```python
from build123d import *

# Parameters (mm, degrees)
SKETCH_1_W          = 35
SKETCH_1_H          = 35
EXTRUDE_1_DEPTH     = 1.6
EXTRUDE_1_2_DEPTH   = 1.6
EXTRUDE_1_3_DEPTH   = 1.6
EXTRUDE_1_4_DEPTH   = 1.6
SKETCH_2_W          = 10
SKETCH_2_H          = 4
SKETCH_2_W_2        = 4
SKETCH_2_H_2        = 10
EXTRUDE_2_DEPTH     = 1.6
CHAMFER_1_SIZE      = 5
FILLET_1_R          = 1
FILLET_2_R          = 2
SKETCH_3_R          = 0.75
CUT_EXTRUDE_1_DEPTH = 105.664033937
SKETCH_4_R          = 0.75
CUT_EXTRUDE_2_DEPTH = 105.664033937


with BuildPart() as part:
    # Sketch 1 → Extrude 1 (new body)
    with BuildSketch(Plane(origin=(0, 0, 0), x_dir=(1, 0, 0), z_dir=(0, 1, 0))):
        with Locations((56.5, -17.5)):
            Rectangle(SKETCH_1_W, SKETCH_1_H)
    extrude(amount=EXTRUDE_1_DEPTH)



with BuildPart() as body_2:
    # Sketch 1 → Extrude 1 2 (new body)
    with BuildSketch(Plane(origin=(0, 0, 0), x_dir=(1, 0, 0), z_dir=(0, 1, 0))):
        with Locations((17.5, -17.5)):
            Rectangle(SKETCH_1_W, SKETCH_1_H)
    extrude(amount=EXTRUDE_1_2_DEPTH)


with BuildPart() as body_3:
    # Sketch 1 → Extrude 1 3 (new body)
    with BuildSketch(Plane(origin=(0, 0, 0), x_dir=(1, 0, 0), z_dir=(0, 1, 0))):
        with Locations((17.5, -56.5)):
            Rectangle(SKETCH_1_W, SKETCH_1_H)
    extrude(amount=EXTRUDE_1_3_DEPTH)


with BuildPart() as body_4:
    # Sketch 1 → Extrude 1 4 (new body)
    with BuildSketch(Plane(origin=(0, 0, 0), x_dir=(1, 0, 0), z_dir=(0, 1, 0))):
        with Locations((56.5, -56.5)):
            Rectangle(SKETCH_1_W, SKETCH_1_H)
    extrude(amount=EXTRUDE_1_4_DEPTH)


with BuildPart() as part_1:
    add(part.part)

    add(body_2.part)  # Extrude 2 merges body 2

    add(body_3.part)  # Extrude 2 merges body 3

    add(body_4.part)  # Extrude 2 merges body 4
    # Sketch 2 → Extrude 2 (add)
    with BuildSketch(Plane(origin=(0, 1.6, 0), x_dir=(1, 0, 0), z_dir=(0, 1, 0))):
        with Locations((15, -37)):
            Rectangle(SKETCH_2_W, SKETCH_2_H)
        with Locations((37, -15)):
            Rectangle(SKETCH_2_W_2, SKETCH_2_H_2)
        with Locations((59, -37)):
            Rectangle(SKETCH_2_W, SKETCH_2_H)
        with Locations((37, -59)):
            Rectangle(SKETCH_2_W_2, SKETCH_2_H_2)
    extrude(amount=-EXTRUDE_2_DEPTH)

    # Chamfer 1
    chamfer_1_edges = [part_1.edges().sort_by_distance(p)[0] for p in [
        (0, 0.8, 39),
        (39, 0.8, 0),
        (39, 0.8, 39),
        (0, 0.8, 0),
    ]]
    chamfer(chamfer_1_edges, length=CHAMFER_1_SIZE)

    # Fillet 1
    fillet_1_edges = [part_1.edges().sort_by_distance(p)[0] for p in [
        (44, 0.8, 39),
        (0, 0.8, 44),
        (5, 0.8, 39),
        (39, 0.8, 5),
        (44, 0.8, 0),
        (0, 0.8, 5),
        (5, 0.8, 0),
        (39, 0.8, 44),
    ]]
    fillet(fillet_1_edges, radius=FILLET_1_R)

    # Fillet 2
    fillet_2_edges = [part_1.edges().sort_by_distance(p)[0] for p in [
        (35, 0.8, 39),
        (0, 0.8, 74),
        (35, 0.8, 74),
        (39, 0.8, 35),
        (74, 0.8, 35),
        (74, 0.8, 0),
        (39, 0.8, 74),
        (74, 0.8, 74),
        (74, 0.8, 39),
        (35, 0.8, 0),
        (35, 0.8, 35),
        (0, 0.8, 35),
    ]]
    fillet(fillet_2_edges, radius=FILLET_2_R)

    # Sketch 3 → Cut-Extrude 1 (cut, through all)
    with BuildSketch(Plane(origin=(0, 1.6, 0), x_dir=(1, 0, 0), z_dir=(0, 1, 0))):
        with Locations(Location((11, -35.5, 0), (0, 0, 270))):
            Circle(SKETCH_3_R)
        with Locations(Location((63, -35.5, 0), (0, 0, 270))):
            Circle(SKETCH_3_R)
        with Locations(Location((63, -38.5, 0), (0, 0, 90))):
            Circle(SKETCH_3_R)
        with Locations(Location((11, -38.5, 0), (0, 0, 90))):
            Circle(SKETCH_3_R)
        with Locations(Location((13, -38.5, 0), (0, 0, 90))):
            Circle(SKETCH_3_R)
        with Locations(Location((13, -35.5, 0), (0, 0, 270))):
            Circle(SKETCH_3_R)
        with Locations(Location((15, -38.5, 0), (0, 0, 90))):
            Circle(SKETCH_3_R)
        with Locations(Location((15, -35.5, 0), (0, 0, 270))):
            Circle(SKETCH_3_R)
        with Locations(Location((17, -38.5, 0), (0, 0, 90))):
            Circle(SKETCH_3_R)
        with Locations(Location((17, -35.5, 0), (0, 0, 270))):
            Circle(SKETCH_3_R)
        with Locations(Location((19, -38.5, 0), (0, 0, 90))):
            Circle(SKETCH_3_R)
        with Locations(Location((19, -35.5, 0), (0, 0, 270))):
            Circle(SKETCH_3_R)
        with Locations(Location((61, -35.5, 0), (0, 0, 270))):
            Circle(SKETCH_3_R)
        with Locations(Location((61, -38.5, 0), (0, 0, 90))):
            Circle(SKETCH_3_R)
        with Locations(Location((59, -35.5, 0), (0, 0, 270))):
            Circle(SKETCH_3_R)
        with Locations(Location((59, -38.5, 0), (0, 0, 90))):
            Circle(SKETCH_3_R)
        with Locations(Location((57, -35.5, 0), (0, 0, 270))):
            Circle(SKETCH_3_R)
        with Locations(Location((57, -38.5, 0), (0, 0, 90))):
            Circle(SKETCH_3_R)
        with Locations(Location((55, -35.5, 0), (0, 0, 270))):
            Circle(SKETCH_3_R)
        with Locations(Location((55, -38.5, 0), (0, 0, 90))):
            Circle(SKETCH_3_R)
    extrude(amount=-CUT_EXTRUDE_1_DEPTH, mode=Mode.SUBTRACT)

    # Sketch 4 → Cut-Extrude 2 (cut, through all)
    with BuildSketch(Plane(origin=(0, 1.6, 0), x_dir=(1, 0, 0), z_dir=(0, 1, 0))):
        with Locations(Location((35.5, -11, 0), (0, 0, 270))):
            Circle(SKETCH_4_R)
        with Locations(Location((38.5, -11, 0), (0, 0, 270))):
            Circle(SKETCH_4_R)
        with Locations(Location((35.5, -13, 0), (0, 0, 270))):
            Circle(SKETCH_4_R)
        with Locations(Location((38.5, -13, 0), (0, 0, 270))):
            Circle(SKETCH_4_R)
        with Locations(Location((35.5, -15, 0), (0, 0, 270))):
            Circle(SKETCH_4_R)
        with Locations(Location((38.5, -15, 0), (0, 0, 270))):
            Circle(SKETCH_4_R)
        with Locations(Location((35.5, -17, 0), (0, 0, 270))):
            Circle(SKETCH_4_R)
        with Locations(Location((38.5, -17, 0), (0, 0, 270))):
            Circle(SKETCH_4_R)
        with Locations(Location((35.5, -19, 0), (0, 0, 270))):
            Circle(SKETCH_4_R)
        with Locations(Location((38.5, -19, 0), (0, 0, 270))):
            Circle(SKETCH_4_R)
        with Locations(Location((35.5, -63, 0), (0, 0, 270))):
            Circle(SKETCH_4_R)
        with Locations(Location((38.5, -63, 0), (0, 0, 270))):
            Circle(SKETCH_4_R)
        with Locations(Location((35.5, -61, 0), (0, 0, 270))):
            Circle(SKETCH_4_R)
        with Locations(Location((38.5, -61, 0), (0, 0, 270))):
            Circle(SKETCH_4_R)
        with Locations(Location((35.5, -59, 0), (0, 0, 270))):
            Circle(SKETCH_4_R)
        with Locations(Location((38.5, -59, 0), (0, 0, 270))):
            Circle(SKETCH_4_R)
        with Locations(Location((35.5, -57, 0), (0, 0, 270))):
            Circle(SKETCH_4_R)
        with Locations(Location((38.5, -57, 0), (0, 0, 270))):
            Circle(SKETCH_4_R)
        with Locations(Location((35.5, -55, 0), (0, 0, 270))):
            Circle(SKETCH_4_R)
        with Locations(Location((38.5, -55, 0), (0, 0, 270))):
            Circle(SKETCH_4_R)
    extrude(amount=-CUT_EXTRUDE_2_DEPTH, mode=Mode.SUBTRACT)


solid = part_1.part
```
Part model, mm, in its own coordinate system. A direction names the side the tool comes from. Round coordinates to 2 decimals unless told otherwise and drop trailing zeros. Write each loop counter-clockwise with the first axis right and the second up, starting at its lowest first coordinate (ties: lowest second). Pieces come first, ordered by that corner, then holes. Notation, with made-up numbers: M 10.5,45.25 L 29.5,45.25 A23 cw 29.5,79.25 Z; hole C -20,79 d6. An arc over 180 degrees is marked long. One line per question, with ' | ' between items.
(1) Saw through at C-C on y = 1.3. Count the separate pieces of the cut face and the enclosed holes in it, then the cut area to 3 significant figures.
Answer key:
separate pieces: 1 | enclosed holes: 41 | area: 4,930 mm^2
(2) Pin check, flat tip, straight feed: pin 1 (0.8 mm diameter, centred on x = 37.5, y = 0.5, fed in from -Z). Stop position of the tip, or through.
Answer key:
pin 1: stops at z = 10
(3) Two-plate mould, pull along X, no slides. Class faces 1 (the face through (8, 1, 39)), 2 (the face through (39, 1, 68)), 3 (the face through (0.57, 0.81, 34.4)): released by +X, released by -X, zero draft, split by the parting line, or undercut.
Answer key:
face 1: zero draft | face 2: undercut | face 3: released by -X
(4) Probe line 1 along Z through (x, y) = (61, 1.35); line 2 along Z through (x, y) = (22.5, 0.55). List the from-to ranges inside material, lowest first.
Answer key:
line 1: z = 0 to 34.75, 36.25 to 37.75, 39.25 to 74 | line 2: z = 0 to 35, 39 to 74
(5) Saw through at B-B on x = 30.5. Write the cut outline in (y, z).
Answer key:
outline: M 0,0 L 1.6,0 L 1.6,35 L 0,35 Z; M 0,39 L 1.6,39 L 1.6,74 L 0,74 Z
(6) 3-axis set-ups, long thin cutter, end or side, ignore diameter. For faces 4 (the face through (39, 1, 27)), 5 (the face through (10, 1, 37)), 6 (the face through (73.4, 0.81, 0.57)), 7 (the face through (64, 1, 37)): which of +Z, -Z, +X, -X, +Y, -Y reach the whole face in a straight line?
Answer key:
face 4: +Y, -Y | face 5: -X, +Y, -Y | face 6: -Z, +X, +Y, -Y | face 7: +X, +Y, -Y
(7) Saw through at A-A on z = 21. Write the cut outline in (x, y), then the cut area to 3 significant figures.
Answer key:
outline: M 0,0 L 35,0 L 35,1.6 L 0,1.6 Z; M 39,0 L 74,0 L 74,1.6 L 39,1.6 Z | area: 112 mm^2
